from build123d import *

# Parameters (mm, degrees)
F1_DEPTH  = 5
F2_W      = 10
F2_H      = 2.5
F3_DEPTH  = 200
F4_W      = 5
F4_H      = 3
F5_DEPTH  = 7.5
F6_W      = 5
F6_H      = 5
F7_DEPTH  = 50
F8_W      = 5
F8_H      = 5
F9_DEPTH  = 50
F12_DEPTH = 5


# Not quite as in the source:
# - a feature names something its author has since deleted; it is built from what else it names


with BuildPart() as f1:
    # F0 (on Top) → F1 (new body)
    with BuildSketch(Plane.XY):
        Polygon((-100, 10), (-100, 0), (-100, -10), (62, -10), (65, -10), (65, -7), (85, -7), (85, -10), (90, -10), (90, 0), (90, 10), (85, 10), (85, 7), (65, 7), (65, 10), (62, 10), align=None)
        Polygon((82.5, 5), (82.5, 0), (82.5, -5), (52.5, -5), (52.5, 0), (52.5, 5), align=None, mode=Mode.SUBTRACT)
        Polygon((65, -10), (62, -10), (62, -13), (90, -13), (90, -10), (85, -10), align=None)
        Polygon((62, 13), (62, 10), (65, 10), (85, 10), (90, 10), (90, 13), align=None)
    extrude(amount=F1_DEPTH)

    # F2 (on face) → F3 (cut)
    with BuildSketch(Plane.YZ.offset(90)):
        with Locations((0, 3.75)):
            Rectangle(F2_W, F2_H)
    extrude(amount=-F3_DEPTH, mode=Mode.SUBTRACT)

    # F4 (on face) → F5 (join)
    with BuildSketch(Plane.XY.offset(5)):
        with Locations((-97.5, 8.5)):
            Rectangle(F4_W, F4_H)
        with Locations((-97.5, -8.5)):
            Rectangle(F4_W, F4_H)
        with Locations((87.5, -8.5)):
            Rectangle(F4_W, F4_H)
        with Locations((87.5, 8.5)):
            Rectangle(F4_W, F4_H)
    extrude(amount=F5_DEPTH)

    # F6 (on face) → F7 (join)
    with BuildSketch(Plane.XZ.offset(10)):
        with Locations((-97.5, 2.5)):
            Rectangle(F6_W, F6_H)
    extrude(amount=F7_DEPTH)

    # F8 (on face) → F9 (join)
    with BuildSketch(Plane(origin=(0, 10, 0), x_dir=(-1, 0, 0), z_dir=(0, 1, 0))):
        with Locations((97.5, 2.5)):
            Rectangle(F8_W, F8_H)
    extrude(amount=F9_DEPTH)

    # F10 (on face) + F11 (on face) → F12 (join)
    with BuildSketch(Plane.XY.offset(5)):
        with BuildLine():
            ThreePointArc((-100, -57.5), (-99.267766953, -59.267766953), (-97.5, -60))
            ThreePointArc((-97.5, -60), (-95.732233047, -59.267766953), (-95, -57.5))
            ThreePointArc((-95, -57.5), (-97.5, -55), (-100, -57.5))
        make_face()
    with BuildSketch(Plane.XY.offset(5)):
        with BuildLine():
            ThreePointArc((-100, 57.5), (-97.5, 55), (-95, 57.5))
            ThreePointArc((-95, 57.5), (-95.732233047, 59.267766953), (-97.5, 60))
            ThreePointArc((-97.5, 60), (-99.267766953, 59.267766953), (-100, 57.5))
        make_face()
    extrude(amount=F12_DEPTH)


solid = f1.part
Model file for the job. Use its own axes, mm. A direction names the side the tool comes from. Coordinates: 2 decimals unless noted, no trailing zeros. Write each loop counter-clockwise with the first axis right and the second up, starting at its lowest first coordinate (ties: lowest second). Pieces come first, ordered by that corner, then holes. Notation, with made-up numbers: (3.5, 55.5) - (10.5, 55.5) arc R33 ccw to (10.5, 94.5) - close; hole circle Ø4 at (86.25, 21). An arc over 180 degrees is marked (long way). Write each question's results on one line, items separated by ' | '. Start each with the question number.
1) Cut at A-A (z = 7.75). Write the cut outline in (x, y), then the cut area to 3 significant figures.
2) Probe line 1 along X through (y, z) = (-8.5, 0.5); line 2 along Y through (x, z) = (-17, 0.75); line 3 along Y through (x, z) = (28, 4). List the from-to ranges inside material, lowest first. Write a range as from..to.
3) Cut at B-B (x = 40). Write the cut outline in (y, z), then the cut area to 3 significant figures.
4) Cut at C-C (y = -34). Write the cut outline in (x, z).
5) Flat gauge pins, fed straight in: P1, Ø2, axis at x = -99.5, y = -58.5, coming from the +Z side; P2, Ø4, axis at x = 86.5, z = 7.5, coming from the +Y side; P3, Ø4, axis at x = 71.5, z = 2, coming from the +Y side; P4, Ø1.5, axis at y = -26.5, z = 6, coming from the -X side. Where does each tip first touch, or does it go through?
6) Mould opens along Y. For faces 1 (the face through (-95, -35, 2)), 2 (the face through (87, -10, 9)), 3 (the face through (-98, 10, 9)) say: pulls with the +Y half, pulls with the -Y half, needs draft (parallel to the pull), parting line crosses it, or undercut.
7) 3-axis set-ups, long thin cutter, end or side, ignore diameter. For faces 4 (the face through (76, 13, 2)), 5 (the face through (87, 10, 9)), 6 (the face through (75, 7, 2)), 7 (the face through (87, -7, 9)): which of +Z, -Z, +X, -X, +Y, -Y reach the whole face in a straight line?
Returned:
1) outline: circle Ø5 at (-97.5, -57.5); (-100, -10) - (-95, -10) - (-95, -7) - (-100, -7) - close; (-100, 7) - (-95, 7) - (-95, 10) - (-100, 10) - close; circle Ø5 at (-97.5, 57.5); (85, -10) - (90, -10) - (90, -7) - (85, -7) - close; (85, 7) - (90, 7) - (90, 10) - (85, 10) - close | area: 99.3 mm^2
2) line 1: -100..65, 85..90 | line 2: -10..10 | line 3: -10..-5, 5..10
3) outline: (-10, 0) - (10, 0) - (10, 5) - (5, 5) - (5, 2.5) - (-5, 2.5) - (-5, 5) - (-10, 5) - close | area: 75.0 mm^2
4) outline: (-100, 0) - (-95, 0) - (-95, 5) - (-100, 5) - close
5) P1: z = 10 | P2: y = 10 | P3: y = 13 | P4: through
6) face 1: needs draft | face 2: pulls with the -Y half | face 3: undercut
7) face 4: +Z, -Z, +X, +Y | face 5: +Z, +X, -X, +Y | face 6: +Z, -Z | face 7: +Z, +X, -X
